Geometry: final body of the model. Coordinates: model frame, mm. Face numbers are marked on the shaded views. Give positions to 0.01 mm unless a question says otherwise; leave off trailing zeros. Loops run counter-clockwise (first coordinate to the right, second up) from the corner with the lowest first, then second, coordinate; pieces in that order, holes last.
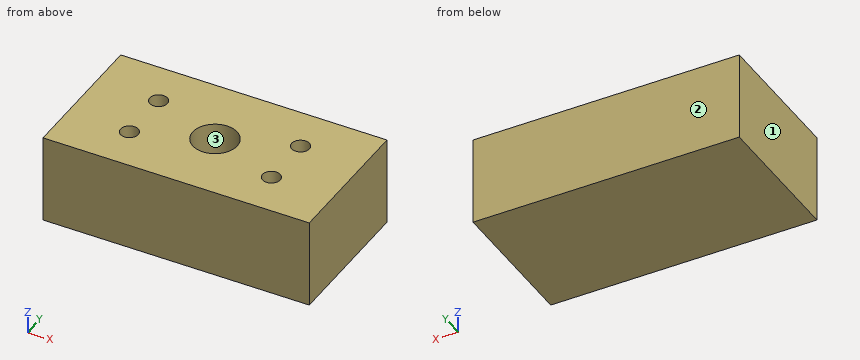
from build123d import *

# Parameters (mm, degrees)
F0_W     = 150
F0_H     = 80
F1_DEPTH = 50
F2_R     = 12.5
F3_DEPTH = 20
F2_R_2   = 5
F4_DEPTH = 10


with BuildPart() as f1:
    # F0 (on Top) → F1 (new body)
    with BuildSketch(Plane.XY):
        with Locations((75, 40)):
            Rectangle(F0_W, F0_H)
    extrude(amount=-F1_DEPTH)

    # F2 (on face) → F3 (cut)
    with BuildSketch(Plane.XY):
        with Locations((75, 40)):
            Circle(F2_R)
    extrude(amount=-F3_DEPTH, mode=Mode.SUBTRACT)

    # F2 (on face) → F4 (cut)
    with BuildSketch(Plane.XY):
        with Locations((35, 55)):
            Circle(F2_R_2)
        with Locations((115, 55)):
            Circle(F2_R_2)
        with Locations((35, 25)):
            Circle(F2_R_2)
        with Locations((115, 25)):
            Circle(F2_R_2)
    extrude(amount=-F4_DEPTH, mode=Mode.SUBTRACT)


solid = f1.part
Item 1: Pin query (flat end, axial travel): pin 1 (5 mm diameter, centred on x = 36.5, y = 55.5, fed in from +Z); pin 2 (8 mm diameter, centred on x = 72.5, z = -42, fed in from -Y); pin 3 (7.5 mm diameter, centred on x = 75, y = 45.5, fed in from +Z). Return the tip coordinate at first contact, or that it passes through.
Values follow:
pin 1: stops at z = -10
pin 2: stops at y = 0
pin 3: stops at z = -20
Item 2: Ray query, probe 1 along Y at (x, z) = (35, -3.5); probe 2 along Z at (x, y) = (114, 21). Return the intervals inside material, ascending.
Values follow:
probe 1: y = 0 to 20, 30 to 50, 60 to 80
probe 2: z = -50 to -10
Item 3: Section query A-A on z = -6.5. Return loops of the section in (x, y), plus the area to 3 significant figures.
Values follow:
outline: (0, 0) - (150, 0) - (150, 80) - (0, 80) - close; hole circle Ø10 at (35, 25); hole circle Ø10 at (35, 55); hole circle Ø25 at (75, 40); hole circle Ø10 at (115, 25); hole circle Ø10 at (115, 55)
area: 11,200 mm2
Item 4: Section query C-C on x = 75. Return loops of the section in (y, z).
Values follow:
outline: (0, -50) - (80, -50) - (80, 0) - (52.5, 0) - (52.5, -20) - (27.5, -20) - (27.5, 0) - (0, 0) - close
Item 5: Draft query along Y for the marked faces 1, 2 and 3. Return one class per face: +Y half, -Y half, draft (parallel to the pull), parting line (faces both ways), or undercut.
Values follow:
face 1: draft
face 2: +Y half
face 3: undercut
Item 6: Section query D-D on z = -17.5. Return loops of the section in (x, y).
Values follow:
outline: (0, 0) - (150, 0) - (150, 80) - (0, 80) - close; hole circle Ø25 at (75, 40)
Item 7: Section query B-B on y = 40. Return loops of the section in (x, z).
Values follow:
outline: (0, -50) - (150, -50) - (150, 0) - (87.5, 0) - (87.5, -20) - (62.5, -20) - (62.5, 0) - (0, 0) - close
